Answer from the drawing. Dimensions are ordinates in mm from the lowest x, y and z of the part. A direction names the side the tool comes from. Round coordinates to 2 decimals unless told otherwise and drop trailing zeros. Loops run counter-clockwise (first coordinate to the right, second up) from the corner with the lowest first, then second, coordinate; pieces in that order, holes last.
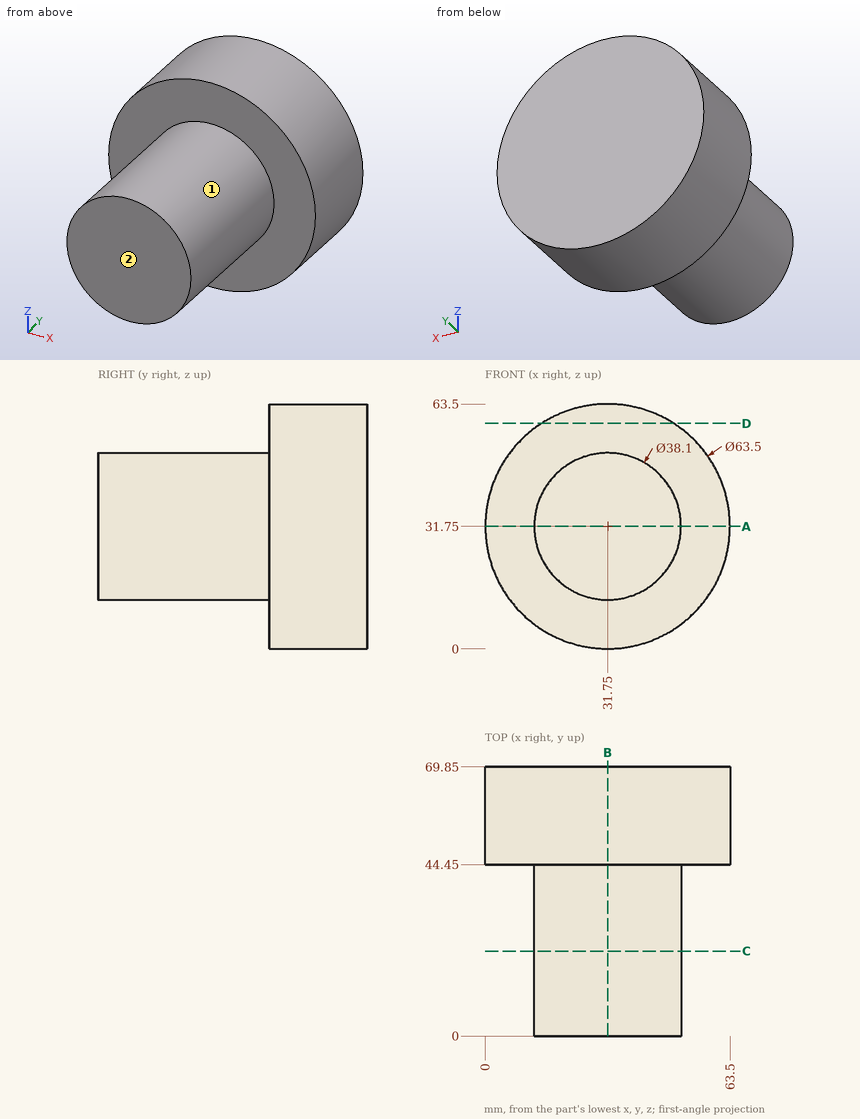
Item 1: Section D-D, the plane z = 58.5 is taken. Give the vertices of the cut face in (x, y).
Item 2: Section B-B, the plane x = 31.75 is taken. Give the vertices of the cut face in (y, z), plus the area to 3 significant figures.
Item 3: For the marked faces 1 and 2, determine the directions among +Z, -Z, +X, -X, +Y, -Y from which every point of the face is accessible in a straight line to the end or side of a thin tool.
Item 4: Each of these flat-tipped pins is pushed along its axis until it touches: P1, Ø2, axis at x = 27, y = 48, coming from the +Z side; P2, Ø10, axis at y = 23, z = 27, coming from the +X side; P3, Ø3, axis at x = 18.5, y = 9.5, coming from the +Z side. Where does it stop, or does it pass through?
Item 5: Section A-A, the plane z = 31.75 is taken. Give the vertices of the cut face in (x, y).
Item 6: Section C-C, the plane y = 22 is taken. Give the vertices of the cut face in (x, z), plus the area to 3 significant figures.
Item 7: Straight lines are drawn through the part: line 1 (Y direction, x = 53, z = 33); line 2 (X direction, y = 51, z = 51); line 3 (Z direction, x = 44.5, y = 44.5). For each, find the intervals that lie inside material, in ascending order.
Answer below:
1. outline: (14.65, 44.45) - (48.85, 44.45) - (48.85, 69.85) - (14.65, 69.85) - close
2. outline: (0, 12.7) - (44.45, 12.7) - (44.45, 0) - (69.85, 0) - (69.85, 63.5) - (44.45, 63.5) - (44.45, 50.8) - (0, 50.8) - close
2. area: 3,310 mm2
3. face 1: -Y
3. face 2: +Z, -Z, +X, -X, -Y
4. P1: stops at z = 63.28
4. P2: stops at x = 50.8
4. P3: stops at z = 46.74
5. outline: (0, 44.45) - (12.7, 44.45) - (12.7, 0) - (50.8, 0) - (50.8, 44.45) - (63.5, 44.45) - (63.5, 69.85) - (0, 69.85) - close
6. outline: circle Ø38.1 at (31.75, 31.75)
6. area: 1,140 mm2
7. line 1: y = 44.45 to 69.85
7. line 2: x = 6.5 to 57
7. line 3: z = 2.67 to 60.83
